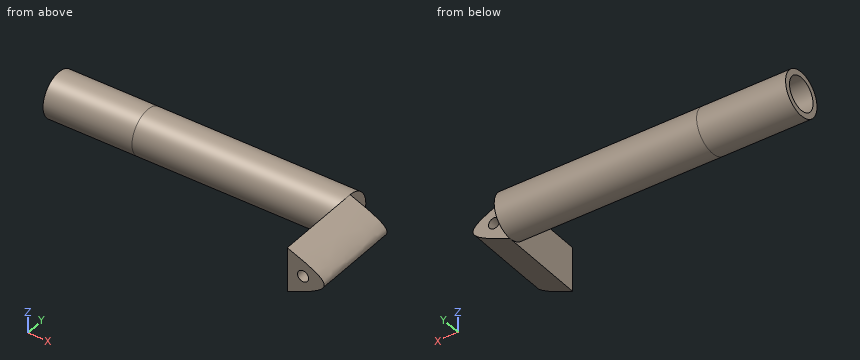
```python
from build123d import *

# Parameters (mm, degrees)
F0_R     = 12.7
F0_R_2   = 9.525
F1_DEPTH = 57.785
F2_R     = 12.7
F3_DEPTH = 2.54
F4_R     = 3.175
F5_DEPTH = 50.8
F6_R     = 12.7
F6_R_2   = 9.525
F7_DEPTH = 50.8


with BuildPart() as f1:
    # F0 (on Right) → F1 (new body, symmetric)
    with BuildSketch(Plane.YZ):
        Circle(F0_R)
        Circle(F0_R_2, mode=Mode.SUBTRACT)
    extrude(amount=F1_DEPTH, both=True)

    # F2 (on face) → F3 (join)
    with BuildSketch(Plane.YZ.offset(57.785)):
        Circle(F2_R)
    extrude(amount=-F3_DEPTH)

    # F4 (on Front) → F5 (join)
    with BuildSketch(Plane.XZ):
        with BuildLine():
            Line((57.785, 12.7), (57.785, 0))
            Line((57.785, 0), (57.785, -12.7))
            add(Edge.make_bspline(
                [(57.785, 12.7), (68.3229282963, 8.4666666667), (89.398784889, 0), (68.3229282963, -8.4666666667), (57.785, -12.7)],
                knots=[0, 0, 0, 0, 0.5, 1, 1, 1, 1], degree=3))
        make_face()
        with Locations((66.7953193188, 0)):
            Circle(F4_R, mode=Mode.SUBTRACT)
    extrude(amount=F5_DEPTH)

    # F6 (on face) → F7 (join)
    with BuildSketch(Plane(origin=(-57.785, 0, 0), x_dir=(0, -1, 0), z_dir=(-1, 0, 0))):
        Circle(F6_R)
        Circle(F6_R_2, mode=Mode.SUBTRACT)
    extrude(amount=F7_DEPTH)


solid = f1.part
```
CAD build for the part. Positions are in the model's coordinates, mm. Coordinates: 2 decimals unless noted, no trailing zeros. Order: outer loops, then holes, each group sorted by start corner. A loop starts at its lowest first (then second) coordinate and runs counter-clockwise, first axis right, second up. Notation, with made-up numbers: (56, 7) - (95, 7) arc R23 cw to (95, 46) - close; hole circle Ø9 at (-24, 0.5). An arc over 180 degrees is marked (long way). Answer in a Markdown table with one row per item.
1. Drill centre lines: L1, parallel to Z at x = 30.5, y = 0 (3 decimals); L2, parallel to Z at x = -98.5, y = 7.5. Where is each one in solid material? Low to high. Write a range as from..to.
Answer:
| item | result |
|---|---|
| L1 | -12.7..-9.525, 9.525..12.7 |
| L2 | -10.25..-5.87, 5.87..10.25 |
2. Flat gauge pins, fed straight in: P1, Ø6.5, axis at x = 72.5, z = 2, coming from the +Y side; P2, Ø12, axis at y = -9, z = -9, coming from the -X side (3 decimals); P3, Ø4, axis at y = 3.5, z = 2.5, coming from the +X side (3 decimals); P4, Ø8, axis at x = -21, z = -8.5, coming from the -Y side. Where does each tip first touch, or does it go through?
Answer:
| item | result |
|---|---|
| P1 | y = 0 |
| P2 | x = -108.585 |
| P3 | x = 57.785 |
| P4 | y = -11.88 |
3. Slice it at A-A, the plane x = -39. List the corners of the cut face in (y, z) (3 decimals).
Answer:
| item | result |
|---|---|
| outline | circle Ø25.4 at (0, 0); hole circle Ø19.05 at (0, 0) |
